```python
from build123d import *

# Parameters (mm, degrees)
SKETCH1_R           = 1.8
SKETCH1_R_2         = 3
BOSS_EXTRUDE1_DEPTH = 4.15
SKETCH2_R           = 4.175
SKETCH2_R_2         = 3
BOSS_EXTRUDE2_DEPTH = 9.65
SKETCH3_R           = 3
CUT_EXTRUDE1_DEPTH  = 2.7


with BuildPart() as part:
    # Sketch1 → Boss-Extrude1 (new body)
    with BuildSketch(Plane(origin=(0, 0, 0), x_dir=(1, 0, 0), z_dir=(0, 1, 0))):
        with BuildLine():
            Line((-9.279008568, -5.575), (9.279008568, -5.575))
            ThreePointArc((9.279008568, -5.575), (10.825, 0), (9.279008568, 5.575))
            Line((9.279008568, 5.575), (-9.279008568, 5.575))
            ThreePointArc((-9.279008568, 5.575), (-10.825, 0), (-9.279008568, -5.575))
        make_face()
        with Locations((-7.5, 0)):
            Circle(SKETCH1_R, mode=Mode.SUBTRACT)
        with Locations((7.5, 0)):
            Circle(SKETCH1_R, mode=Mode.SUBTRACT)
        Circle(SKETCH1_R_2, mode=Mode.SUBTRACT)
    extrude(amount=BOSS_EXTRUDE1_DEPTH)

    # Sketch2 → Boss-Extrude2 (add)
    with BuildSketch(Plane(origin=(0, 4.15, 0), x_dir=(1, 0, 0), z_dir=(0, 1, 0))):
        Circle(SKETCH2_R)
        Circle(SKETCH2_R_2, mode=Mode.SUBTRACT)
    extrude(amount=BOSS_EXTRUDE2_DEPTH)

    # Sketch3 → Cut-Extrude1 (cut)
    with BuildSketch(Plane.XZ):
        with Locations((7.5, 0)):
            Circle(SKETCH3_R)
        with Locations((-7.5, 0)):
            Circle(SKETCH3_R)
    extrude(amount=-CUT_EXTRUDE1_DEPTH, mode=Mode.SUBTRACT)


solid = part.part
```
Geometry: final body of the model. Coordinates: model frame, mm. A direction names the side the tool comes from. Give positions to 0.01 mm unless a question says otherwise; leave off trailing zeros. Write each loop counter-clockwise with the first axis right and the second up, starting at its lowest first coordinate (ties: lowest second). Pieces come first, ordered by that corner, then holes.
1. Section query D-D, the plane x = 0. Return loops of the section in (y, z) (3 decimals), then the cut area to 4 significant figures.
2. Pin query (flat end, axial travel): P1, Ø5.5, axis at x = -7.5, z = 0, coming from the +Y side; P2, Ø5.5, axis at x = 7.5, z = 0, coming from the -Y side; P3, Ø1.5, axis at y = 6, z = 0, coming from the +X side (3 decimals). Return the tip coordinate at first contact, or that it passes through.
3. Section query A-A, the plane x = -7.5. Return loops of the section in (y, z) (3 decimals).
4. Draft query along Z for faces 4 (the cylindrical face through (-4.73, 1.33, -1.15)), 5 (the cylindrical face through (10.825, 2.046, 0.082)), 6 (the flat face through (2, 4.15, -4)), 7 (the flat face through (0, 2, 5.575)). Return one class per face: released by +Z, released by -Z, zero draft, split by the parting line, or undercut.
5. Section query C-C, the plane z = -2.75. Return loops of the section in (x, y), then the cut area to 3 significant figures.
6. Section query B-B, the plane y = 2. Return loops of the section in (x, z) (3 decimals), then the cut area to 3 significant figures.
7. Line query: probe 1 along Z at (x, y) = (-7.5, 3.2) (3 decimals); probe 2 along X at (y, z) = (6, 0) (3 decimals); probe 3 along X at (y, z) = (3.1, 0) (3 decimals). Output: solid intervals per line, ascending.
8. Reachability of faces 1 (the cylindrical face through (3.982, 8.907, -1.254)), 2 (the cylindrical face through (10.27, 1.33, -1.15)), 3 (the flat face through (2, 0, -3)) from +Z, -Z, +X, -X, +Y, -Y: full face, straight path, thin tool, end or side. Return the list, or none.
Computed:
1. outline: (0, -5.575) - (4.15, -5.575) - (4.15, -4.175) - (13.8, -4.175) - (13.8, -3) - (0, -3) - close; (0, 3) - (13.8, 3) - (13.8, 4.175) - (4.15, 4.175) - (4.15, 5.575) - (0, 5.575) - close
1. area: 44.05 mm2
2. P1: stops at y = 4.15
2. P2: stops at y = 2.7
2. P3: stops at x = 4.175
3. outline: (0, -5.575) - (4.15, -5.575) - (4.15, -1.8) - (2.7, -1.8) - (2.7, -3) - (0, -3) - close; (0, 3) - (2.7, 3) - (2.7, 1.8) - (4.15, 1.8) - (4.15, 5.575) - (0, 5.575) - close
4. face 4: undercut
4. face 5: split by the parting line
4. face 6: zero draft
4. face 7: released by +Z
5. outline: (-10.47, 0) - (-8.7, 0) - (-8.7, 2.7) - (-6.3, 2.7) - (-6.3, 0) - (-1.2, 0) - (-1.2, 13.8) - (-3.14, 13.8) - (-3.14, 4.15) - (-10.47, 4.15) - close; (1.2, 0) - (6.3, 0) - (6.3, 2.7) - (8.7, 2.7) - (8.7, 0) - (10.47, 0) - (10.47, 4.15) - (3.14, 4.15) - (3.14, 13.8) - (1.2, 13.8) - close
5. area: 101 mm2
6. outline: (-9.279, -5.575) - (9.279, -5.575) arc R10.825 ccw to (9.279, 5.575) - (-9.279, 5.575) arc R10.825 ccw to start; hole circle Ø6 at (-7.5, 0); hole circle Ø6 at (0, 0); hole circle Ø6 at (7.5, 0)
6. area: 145 mm2
7. probe 1: z = -5.575 to -1.8, 1.8 to 5.575
7. probe 2: x = -4.175 to -3, 3 to 4.175
7. probe 3: x = -10.825 to -9.3, -5.7 to -3, 3 to 5.7, 9.3 to 10.825
8. face 1: +Y
8. face 2: -Y
8. face 3: +Z, -Z, +X, -X, -Y
